Check sheet for the modelled part. Datum: model origin and axes. Units: mm. Face numbers are marked on the shaded views. A direction names the side the tool comes from. Coordinates: 2 decimals unless noted, no trailing zeros. Loops run counter-clockwise (first coordinate to the right, second up) from the corner with the lowest first, then second, coordinate; pieces in that order, holes last. Notation, with made-up numbers: (73.5, 75) - (80.5, 75) arc R16 ccw to (80.5, 90) - close; hole circle Ø2 at (-14.75, -39.5). An arc over 180 degrees is marked (long way). Write each question's results on one line, items separated by ' | '. Start each with the question number.
1. Cross-section at A-A (x = 0). Record the cut outline in (y, z).
2. Thickness scan on line 1 (Z direction, x = 0, y = 8); line 2 (X direction, y = 4.75, z = 24.5); line 3 (Z direction, x = -7, y = 7.5). Record the ranges inside material, lowest first. Write a range as [from, to].
3. Gauge pin test, flat ends, axial feed: P1, Ø2, axis at x = 7, z = 64, coming from the -Y side; P2, Ø1.5, axis at y = 6, z = 90.5, coming from the -X side (3 decimals); P3, Ø3, axis at y = 5, z = 98.15, coming from the +X side; P4, Ø5, axis at y = 4, z = 45, coming from the +X side. Record the tip position at first contact, or that the pin passes through.
4. Cross-section at B-B (z = 42). Record the cut outline in (x, y), and give its area (3 significant figures).
5. Cross-section at D-D (x = 18). Record the cut outline in (y, z).
6. Draft check along X on the marked faces 4, 5 and 6. Enter one of: released by +X, released by -X, zero draft, split by the parting line, or undercut.
7. Cross-section at C-C (y = 1.75). Record the cut outline in (x, z), and give its area (3 significant figures).
8. Tool access check on the marked faces 1, 2 and 3. Record the directions out of +Z, -Z, +X, -X, +Y, -Y that give a thin tool (end or side, any length) a straight path to the whole face; none if there is none.
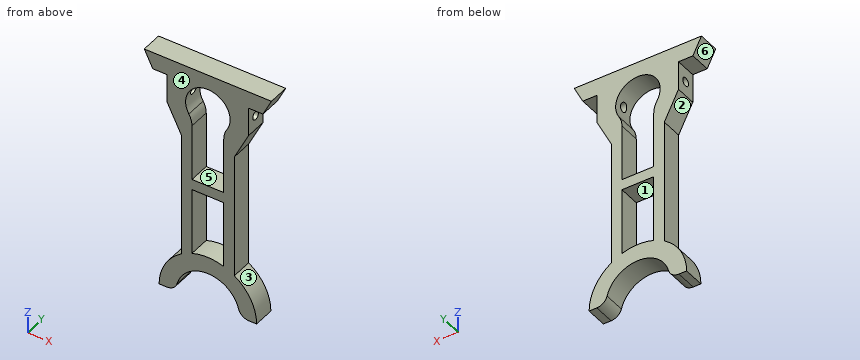
```python
from build123d import *

# Parameters (mm, degrees)
BOSS_EXTRUDE1_DEPTH = 10
FILLET1_R           = 10
FILLET2_R           = 5
CUT_EXTRUDE1_DEPTH  = 10
SKETCH7_R           = 2
CUT_EXTRUDE2_DEPTH  = 43
SKETCH8_W           = 15
SKETCH8_H           = 5
BOSS_EXTRUDE3_DEPTH = 10


with BuildPart() as part:
    # Sketch1 → Boss-Extrude1 (new body)
    with BuildSketch(Plane(origin=(0, 0, 0), x_dir=(1, 0, 0), z_dir=(0, 1, 0))):
        with BuildLine():
            Line((12.5, -23), (12.5, -19.306734576))
            ThreePointArc((12.5, -19.306734576), (20.205197351, -10.988630488), (23, 0))
            Line((23, 0), (15, 0))
            ThreePointArc((15, 0), (0, -15), (-15, 0))
            Line((-15, 0), (-23, 0))
            ThreePointArc((-23, 0), (-20.205197351, -10.988630488), (-12.5, -19.306734576))
            Line((-12.5, -19.306734576), (-12.5, -23))
            Line((-12.5, -23), (-12.5, -78))
            Line((-12.5, -78), (-30, -113))
            Line((-30, -113), (-12.5, -113))
            Line((-12.5, -113), (12.5, -113))
            Line((12.5, -113), (30, -113))
            Line((30, -113), (12.5, -78))
            Line((12.5, -78), (12.5, -23))
        make_face()
        with BuildLine():
            ThreePointArc((-7.5, -88.04908974), (0, -105.897558969), (7.5, -88.04908974))
            Line((7.5, -88.04908974), (7.5, -33.180945535))
            Line((7.5, -33.180945535), (7.5, -21.742814905))
            ThreePointArc((7.5, -21.742814905), (0, -23), (-7.5, -21.742814905))
            Line((-7.5, -21.742814905), (-7.5, -33.180945535))
            Line((-7.5, -33.180945535), (-7.5, -88.04908974))
        make_face(mode=Mode.SUBTRACT)
    extrude(amount=BOSS_EXTRUDE1_DEPTH)

    # Fillet1
    fillet1_edges = [part.edges().sort_by_distance(p)[0] for p in [
        (7.5, 5, 88.04908974),
        (-7.5, 5, 88.04908974),
    ]]
    fillet(fillet1_edges, radius=FILLET1_R)

    # Fillet2
    fillet2_edges = [part.edges().sort_by_distance(p)[0] for p in [
        (-15, 5, 0),
        (15, 5, 0),
    ]]
    fillet(fillet2_edges, radius=FILLET2_R)

    # Sketch6 → Cut-Extrude1 (cut)
    with BuildSketch(Plane(origin=(0, 10, 0), x_dir=(1, 0, 0), z_dir=(0, 1, 0))):
        Polygon((25.97702769, -104.95405538), (19.174519353, -91.349038706), (19.174519353, -104.95405538), align=None)
        Polygon((-19.174519353, -104.95405538), (-19.174519353, -91.349038706), (-25.97702769, -104.95405538), align=None)
    extrude(amount=-CUT_EXTRUDE1_DEPTH, mode=Mode.SUBTRACT)

    # Sketch7 → Cut-Extrude2 (cut)
    with BuildSketch(Plane(origin=(19.174519353, 0, 0), x_dir=(0, 0, -1), z_dir=(1, 0, 0))):
        with Locations((-98.151547043, 5)):
            Circle(SKETCH7_R)
    extrude(amount=-CUT_EXTRUDE2_DEPTH, mode=Mode.SUBTRACT)

    # Sketch8 → Boss-Extrude3 (add)
    with BuildSketch(Plane(origin=(0, 10, 0), x_dir=(1, 0, 0), z_dir=(0, 1, 0))):
        with Locations((0, -55.731647811)):
            Rectangle(SKETCH8_W, SKETCH8_H)
    extrude(amount=-BOSS_EXTRUDE3_DEPTH)


solid = part.part
```
Established:
1) outline: (0, 15) - (10, 15) - (10, 23) - (0, 23) - close; (0, 53.23) - (10, 53.23) - (10, 58.23) - (0, 58.23) - close; (0, 105.9) - (10, 105.9) - (10, 113) - (0, 113) - close
2) line 1: [15, 23], [53.23, 58.23], [105.9, 113] | line 2: [-12.5, -7.5], [7.5, 12.5] | line 3: [13.27, 21.91], [53.23, 58.23], [103.22, 113]
3) P1: y = 0 | P2: x = -19.125 | P3: through | P4: x = 12.5
4) outline: (-12.5, 0) - (-7.5, 0) - (-7.5, 10) - (-12.5, 10) - close; (7.5, 0) - (12.5, 0) - (12.5, 10) - (7.5, 10) - close | area: 100 mm^2
5) outline: (0, 0.19) - (10, 0.19) - (10, 14.32) - (0, 14.32) - close; (0, 89) - (10, 89) - (10, 113) - (0, 113) - close; hole circle Ø4 at (5, 98.15)
6) face 4: zero draft | face 5: undercut | face 6: released by -X
7) outline: (-30, 113) - (-25.98, 104.95) - (-19.17, 104.95) - (-19.17, 91.35) - (-12.5, 78) - (-12.5, 19.31) arc R23 ccw to (-23, 0) - (-19.36, 0) arc R5 ccw to (-14.52, 3.75) arc R15 cw to (14.52, 3.75) arc R5 ccw to (19.36, 0) - (23, 0) arc R23 ccw to (12.5, 19.31) - (12.5, 78) - (19.17, 91.35) - (19.17, 104.95) - (25.98, 104.95) - (30, 113) - close; hole (-8.96, 89.93) arc R10 cw to (-7.5, 84.72) - (-7.5, 58.23) - (7.5, 58.23) - (7.5, 84.72) arc R10 cw to (8.96, 89.93) arc R10.5 ccw (long way) to start; hole (-7.5, 21.74) arc R23 cw to (7.5, 21.74) - (7.5, 53.23) - (-7.5, 53.23) - close | area: 2,050 mm^2
8) face 1: +Y, -Y | face 2: -X, +Y, -Y | face 3: +X, +Y, -Y
